CAD build for the part. Positions are in the model's coordinates, mm. Face numbers are marked on the shaded views. A direction names the side the tool comes from. Round coordinates to 2 decimals unless told otherwise and drop trailing zeros. Loops run counter-clockwise (first coordinate to the right, second up) from the corner with the lowest first, then second, coordinate; pieces in that order, holes last.
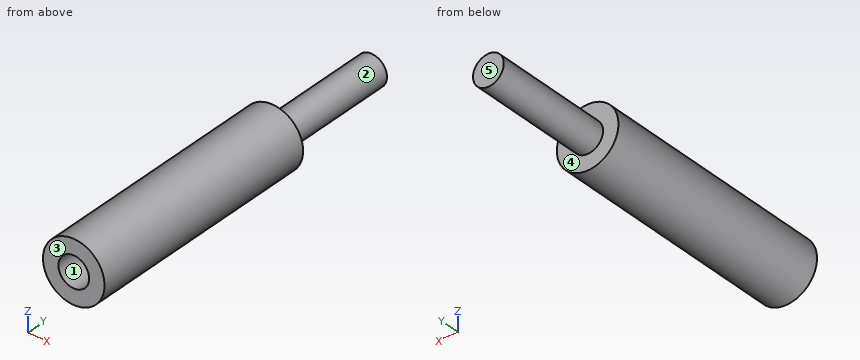
```python
from build123d import *

# Parameters (mm, degrees)
SKETCH1_R                        = 3.175
BOSS_EXTRUDE1_DEPTH              = 25.4
SKETCH2_R                        = 1.5875
BOSS_EXTRUDE2_DEPTH              = 12.7
F_1_8_0_125_DIAMETER_HOLE1_D     = 3.175
F_1_8_0_125_DIAMETER_HOLE1_DEPTH = 12.7
F_1_8_0_125_DIAMETER_HOLE1_TIP   = 0.953866233


with BuildPart() as part:
    # Sketch1 → Boss-Extrude1 (new body)
    with BuildSketch(Plane(origin=(0, 0, 0), x_dir=(1, 0, 0), z_dir=(0, 1, 0))):
        with Locations(Location((0, 0, 0), (0, 0, 270))):
            Circle(SKETCH1_R)
    extrude(amount=BOSS_EXTRUDE1_DEPTH)

    # Sketch2 → Boss-Extrude2 (add)
    with BuildSketch(Plane(origin=(0, 25.4, 0), x_dir=(1, 0, 0), z_dir=(0, 1, 0))):
        with Locations(Location((0, 0, 0), (0, 0, 270))):
            Circle(SKETCH2_R)
    extrude(amount=BOSS_EXTRUDE2_DEPTH)

    # 1/8 (0.125) Diameter Hole1
    with Locations(Plane.XZ):
        with Locations((0, 0)):
            Hole(F_1_8_0_125_DIAMETER_HOLE1_D / 2, depth=F_1_8_0_125_DIAMETER_HOLE1_DEPTH)
            with Locations((0, 0, -(F_1_8_0_125_DIAMETER_HOLE1_DEPTH + F_1_8_0_125_DIAMETER_HOLE1_TIP / 2))):  # 118° drill point
                Cone(0, F_1_8_0_125_DIAMETER_HOLE1_D / 2, F_1_8_0_125_DIAMETER_HOLE1_TIP, mode=Mode.SUBTRACT)


solid = part.part
```
Item 1: Cut at C-C, the plane x = -2.5. Give the cut face in (y, z), plus the area to 3 significant figures.
Answers follow:
outline: (0, -1.96) - (25.4, -1.96) - (25.4, 1.96) - (0, 1.96) - close
area: 99.4 mm2
Item 2: Probe line 1 (X direction, y = 3.5, z = 0) (1 decimal); line 2 (Y direction, x = 1.5, z = 2); line 3 (X direction, y = 7.5, z = -0.5). List the from-to ranges inside material, lowest first.
Answers follow:
line 1: x = -3.2 to -1.6, 1.6 to 3.2
line 2: y = 0 to 25.4
line 3: x = -3.14 to -1.51, 1.51 to 3.14
Item 3: Cut at D-D, the plane y = 31. Give the cut face in (x, z) (1 decimal).
Answers follow:
outline: circle Ø3.2 at (0, 0)
Item 4: Two-plate mould, pull along X, no slides. Class the marked faces 1, 2 and 3: released by +X, released by -X, zero draft, split by the parting line, or undercut.
Answers follow:
face 1: undercut
face 2: split by the parting line
face 3: zero draft
Item 5: Cut at B-B, the plane y = 25. Give the cut face in (x, z) (3 decimals), plus the area to 3 significant figures.
Answers follow:
outline: circle Ø6.35 at (0, 0)
area: 31.7 mm2
Item 6: Flat gauge pin, fed straight in: P1, Ø1.5, axis at x = 2.5, y = 12.5, coming from the -Z side. Where does the tip first touch, or does it go through?
Answers follow:
P1: stops at z = -2.65
Item 7: 3-axis set-ups, long thin cutter, end or side, ignore diameter. For the marked faces 4 and 5: which of +Z, -Z, +X, -X, +Y, -Y reach the whole face in a straight line?
Answers follow:
face 4: +Y
face 5: +Z, -Z, +X, -X, +Y
